Input: part model. Units: mm. Frame: model coordinates. Face numbers are marked on the shaded views. A direction names the side the tool comes from. Give positions to 0.01 mm unless a question says otherwise; leave off trailing zeros. Write each loop counter-clockwise with the first axis right and the second up, starting at its lowest first coordinate (ties: lowest second). Pieces come first, ordered by that corner, then holes. Notation, with made-up numbers: (-16.75, 10.5) -> (14.25, 10.5) arc R16 cw to (14.25, 29.5) -> close; hole circle Ø2 at (69.25, -16). An arc over 180 degrees is marked (long way). Return JSON: item names as keys, results as strings. Group by question number.
Item 1: Line query: line 1 (Y direction, x = 2.25, z = 31.75) (1 decimal); line 2 (X direction, y = -3.25, z = 29) (3 decimals); line 3 (Z direction, x = 7.5, y = -1.5). Output: solid intervals per line, ascending. Write a range as [from, to].
Item 2: Pin query (flat end, axial travel): P1, Ø12, axis at x = 14.5, z = 43.5, coming from the -Y side; P2, Ø1.3, axis at x = 17, y = -0.5, coming from the -Z side; P3, Ø1, axis at x = 4.5, y = -3, coming from the +Z side; P4, Ø1.5, axis at y = -2.5, z = 67.5, coming from the -X side. Return the tip coordinate at first contact, or that it passes through.
Item 3: Section C-C, the plane z = 43.5. Return loops of the section in (x, y) (1 decimal), then the cut area to 3 significant figures.
Item 4: Section A-A, the plane z = 31.75. Return loops of the section in (x, y) (1 decimal).
Item 5: Section D-D, the plane x = -1.75. Return loops of the section in (y, z), then the cut area to 3 significant figures.
Item 6: Set-up query: the marked faces 1 and 2. Return all of +Z, -Z, +X, -X, +Y, -Y with unobstructed straight access to the full face (end or side cutting, diameter ignored); none if empty.
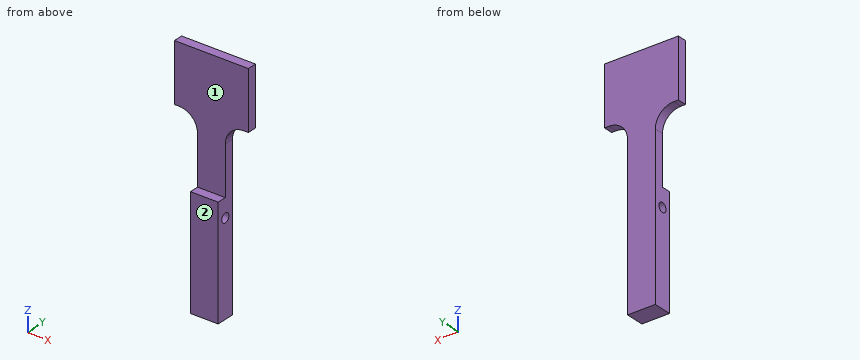
from build123d import *

# Parameters (mm, degrees)
SKETCH1_R           = 1.5875
BOSS_EXTRUDE1_DEPTH = 9.525
SKETCH3_W           = 15
SKETCH3_H           = 3.175
SKETCH3_W_2         = 5
BOSS_EXTRUDE2_DEPTH = 12.7
FILLET1_R           = 6.35


with BuildPart() as part:
    # Sketch1 → Boss-Extrude1 (new body)
    with BuildSketch(Plane(origin=(0, 0, 0), x_dir=(0, 0, -1), z_dir=(1, 0, 0))):
        Polygon((0, -1.5875), (0, 1.5875), (-76.2, 1.5875), (-76.2, -1.5875), (-38.1, -1.5875), (-38.1, -4.7625), (-25.4, -4.7625), (0, -4.7625), align=None)
        with Locations((-31.75, -1.5875)):
            Circle(SKETCH1_R, mode=Mode.SUBTRACT)
        Polygon((0, -1.5875), (0, 1.5875), (-76.2, 1.5875), (-76.2, -1.5875), (-38.1, -1.5875), (-38.1, -4.7625), (-25.4, -4.7625), (0, -4.7625), align=None)
        with Locations((-31.75, -1.5875)):
            Circle(SKETCH1_R, mode=Mode.SUBTRACT)
    extrude(amount=BOSS_EXTRUDE1_DEPTH)

    # Sketch3 → Boss-Extrude2 (add, symmetric)
    with BuildSketch(Plane(origin=(4.7625, 0, 0), x_dir=(0, 0, -1), z_dir=(1, 0, 0))):
        with Locations((-68.7, 0)):
            Rectangle(SKETCH3_W, SKETCH3_H)
        with Locations((-78.7, 0)):
            Rectangle(SKETCH3_W_2, SKETCH3_H)
    extrude(amount=BOSS_EXTRUDE2_DEPTH, both=True)

    # Fillet1
    fillet1_edges = [part.edges().sort_by_distance(p)[0] for p in [
        (0, 0, 61.2),
        (9.525, 0, 61.2),
    ]]
    fillet(fillet1_edges, radius=FILLET1_R)


solid = part.part
Answer below:
{
 "1": {"line 1": "y = [-4.8, -3.2], [0, 1.6]", "line 2": "x = [0, 9.525]", "line 3": "z = [0, 30.16], [33.34, 81.2]"},
 "2": {"P1": "stops at y = -1.59", "P2": "stops at z = 61.2", "P3": "stops at z = 38.1", "P4": "passes through"},
 "3": {"outline": "(0, -1.6) -> (9.5, -1.6) -> (9.5, 1.6) -> (0, 1.6) -> close", "area": "30.2 mm2"},
 "4": {"outline": "(0, -4.8) -> (9.5, -4.8) -> (9.5, -3.2) -> (0, -3.2) -> close; (0, 0) -> (9.5, 0) -> (9.5, 1.6) -> (0, 1.6) -> close"},
 "5": {"outline": "(-1.59, 59.23) -> (1.59, 59.23) -> (1.59, 81.2) -> (-1.59, 81.2) -> close", "area": "69.8 mm2"},
 "6": {"face 1": "+Z, +X, -X, -Y", "face 2": "+Z, -Z, +X, -X, -Y"}
}
